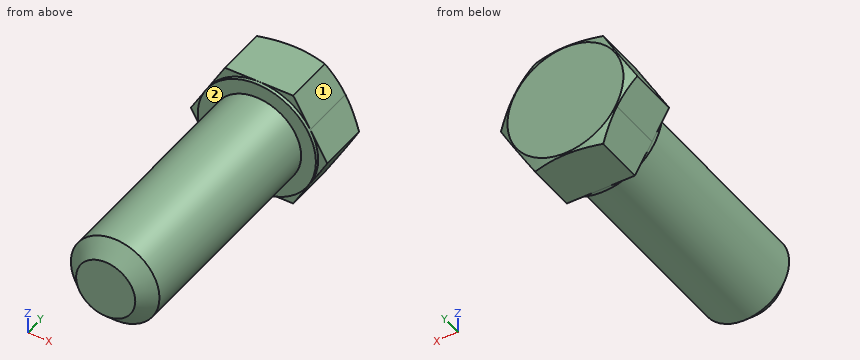
Autodesk Inventor part; units mm, degrees
ref_plane "YZ Plane" through (0, 0, 0) normal (1, 0, 0) x (0, 1, 0)
ref_plane "XZ Plane" through (0, 0, 0) normal (0, 1, 0) x (-1, 0, 0)
ref_plane "XY Plane" through (0, 0, 0) normal (0, 0, 1) x (1, 0, 0)
sketch "Sketch1" plane through (0, 0, 0) normal (0, 0, 1) x (1, 0, 0)
  line L0 (0, 0) -> (9.525, 0)
  line L1 (9.525, 0) -> (9.525, -50.8)
  line L2 (9.525, -50.8) -> (0, -50.8)
  line L3 (0, -50.8) -> (0, 0)
  dimension "d0" = 19.05
  dimension "d1" = 50.8
revolve "Revolution1" add sketch "Sketch1" angle 360 about axis through (0, -50.8, 0) along (0, 1, 0)
chamfer "Chamfer1" distance 3.175 angle 45 1 edges at (-9.525, -50.8, 0)
sketch "Sketch2" plane through (0, 0, 0) normal (0, 1, 0) x (1, 0, 0)
  circle A0 centre (0, 0) radius 12.7
  dimension "d6" = 25.4
extrude "Extrusion1" add sketch "Sketch2" along normal blind 12.7
sketch "Sketch3" plane through (0, 12.7, 0) normal (0, 1, 0) x (1, 0, 0)
  line L0 (14.6647, 0) -> (7.3323, -12.7)
  line L1 (7.3323, -12.7) -> (-7.3323, -12.7)
  line L2 (-7.3323, -12.7) -> (-14.6647, 0)
  line L3 (-14.6647, 0) -> (-7.3323, 12.7)
  line L4 (-7.3323, 12.7) -> (7.3323, 12.7)
  line L5 (7.3323, 12.7) -> (14.6647, 0)
  circle A0 centre (0, 0) radius 12.7 construction
  point P0 (0, 0)
  point P1 (0, 0)
extrude "Extrusion2" add sketch "Sketch3" against normal blind 11.938
sketch "Sketch4" plane through (0, 0, 0) normal (0, 0, 1) x (1, 0, 0)
  line L0 (12.465, 12.7) -> (14.6647, 12.7)
  line L1 (14.6647, 12.7) -> (14.6647, 11.43)
  line L2 (14.6647, 11.43) -> (12.465, 12.7)
  line L3 (0, -0.2588) -> (0, 1.5529)
  line L4 (7.3323, 0) -> (14.6647, 0) construction
  line L5 (7.3323, 12.7) -> (14.6647, 12.7) construction
  line L6 (7.3323, 12.7) -> (7.3323, 0.762) construction
  line L7 (14.6647, 12.7) -> (14.6647, 0.762) construction
  line L8 (14.6647, 12.7) -> (7.3323, 12.7)
  line L9 (10.9985, 0.762) -> (14.6647, 0.762)
  line L10 (7.3323, 0.762) -> (10.9985, 0.762)
  point P0 (0, 0)
  point P1 (16.2522, 7.9375)
  dimension "d11" = 30
  dimension "d17" = 1.27
revolve "Revolution2" cut sketch "Sketch4" angle 360 about axis through (0, -10, 0) along (0, 1, 0)
thread "Thread2"
equation "\"diameter\" = 1.8542"
equation "\"length\" = 19.05"
properties part number "Hinge Pin" material "Steel, Carbon"
Input: part model. Units: mm. Frame: model coordinates. Face numbers are marked on the shaded views. A direction names the side the tool comes from. Give positions to 0.01 mm unless a question says otherwise; leave off trailing zeros. Order: outer loops, then holes, each group sorted by start corner. A loop starts at its lowest first (then second) coordinate and runs counter-clockwise, first axis right, second up.
1. Pin query (flat end, axial travel): pin 1 Ø6 at (x, y) = (0, -24.5) entering from -Z (3 decimals); pin 2 Ø8 at (y, z) = (-22, 2) entering from +X (3 decimals); pin 3 Ø8 at (x, y) = (-11.5, -16.5) entering from +Z. Return the tip coordinate at first contact, or that it passes through.
Computed:
pin 1: stops at z = -9.525
pin 2: stops at x = 9.525
pin 3: stops at z = 5.87
2. Cut plane A-A (y = -44.5). Return loops of the section in (x, z) (3 decimals).
Computed:
outline: circle Ø19.05 at (0, 0)
3. Line query: probe 1 along Z at (x, y) = (-0.25, -11); probe 2 along Y at (x, z) = (-9.5, -5.5); probe 3 along X at (y, z) = (1, 0.75). Output: solid intervals per line, ascending.
Computed:
probe 1: z = -9.52 to 9.52
probe 2: y = 0 to 12.7
probe 3: x = -14.23 to 14.23
4. Set-up query: the marked faces 1 and 2. Return all of +Z, -Z, +X, -X, +Y, -Y with unobstructed straight access to the full face (end or side cutting, diameter ignored); none if empty.
Computed:
face 1: +Z, +X, +Y, -Y
face 2: -Y
